Design review of the part built by this model. Coordinates are the model's own, in mm. Give positions to 0.01 mm unless a question says otherwise; leave off trailing zeros. Loops run counter-clockwise (first coordinate to the right, second up) from the corner with the lowest first, then second, coordinate; pieces in that order, holes last.
from build123d import *

# Parameters (mm, degrees)
SKETCH_1_W             = 0.8
SKETCH_1_H             = 15
EXTRUDE_1_DEPTH        = 203
SKETCH_2_R             = 2.5
SKETCH_3_R             = 1.5
CUT_EXTRUDE_1_DEPTH    = 407.407738607
SKETCH_10_W            = 33
SKETCH_10_H            = 6
CUT_EXTRUDE_4_DEPTH    = 60
PATTERN_LINEAR_1_COUNT = 8
PATTERN_LINEAR_1_PITCH = 50


with BuildPart() as part:
    # 草图1 → 拉伸-薄壁1 (new, symmetric)
    with BuildSketch(Plane.XY):
        with Locations((0.4, 7.5)):
            Rectangle(SKETCH_1_W, SKETCH_1_H)
    extrude(amount=EXTRUDE_1_DEPTH, both=True)

    # 扫描1: sweep along a curve in space
    with BuildLine() as sweep_1_path:
        Line((0.8, 15, 203), (0.8, 15, -203))
    # 草图2 → 扫描1 (sweep)
    with BuildSketch(Plane.XY.offset(203)):
        with Locations((2.5, 15)):
            Circle(SKETCH_2_R)
    sweep(path=sweep_1_path.line)

    # 草图3 → 切除-拉伸1 (cut, through all)
    with BuildSketch(Plane.XY.offset(203)):
        with Locations((2.5, 15)):
            Circle(SKETCH_3_R)
    extrude(amount=-CUT_EXTRUDE_1_DEPTH, mode=Mode.SUBTRACT)

    # 草图10 → 切除-拉伸4 (cut, symmetric)
    with BuildSketch(Plane(origin=(0.8, 0, 0), x_dir=(0, 0, -1), z_dir=(1, 0, 0))):
        with Locations((-165, 15)):
            Rectangle(SKETCH_10_W, SKETCH_10_H)
        with Locations((-99, 15)):
            Rectangle(SKETCH_10_W, SKETCH_10_H)
        with Locations((-33, 15)):
            Rectangle(SKETCH_10_W, SKETCH_10_H)
        with Locations((33, 15)):
            Rectangle(SKETCH_10_W, SKETCH_10_H)
        with Locations((99, 15)):
            Rectangle(SKETCH_10_W, SKETCH_10_H)
        with Locations((165, 15)):
            Rectangle(SKETCH_10_W, SKETCH_10_H)
    extrude(amount=CUT_EXTRUDE_4_DEPTH, both=True, mode=Mode.SUBTRACT)

    # 草图12 → M3 锥坑平头螺钉的锥形沉头孔2 (revolve, cut)
    with BuildSketch(Plane(origin=(0.8, 5.5, -175), x_dir=(0, 0, -1), z_dir=(0, 1, 0))):
        Polygon((0, 0), (0, 0.8), (1.7, 0.8), (1.7, 1.45), (3.15, 0), align=None)
    hole_wizard_m3_2 = revolve(axis=Axis((7.15, 5.5, -175), (-1, 0, 0)), mode=Mode.SUBTRACT)

    # 阵列(线性)1: M3 锥坑平头螺钉的锥形沉头孔2 ×8
    with Locations(*[(0, 0, i * PATTERN_LINEAR_1_PITCH) for i in range(1, PATTERN_LINEAR_1_COUNT)]):
        add(hole_wizard_m3_2, mode=Mode.SUBTRACT)


solid = part.part
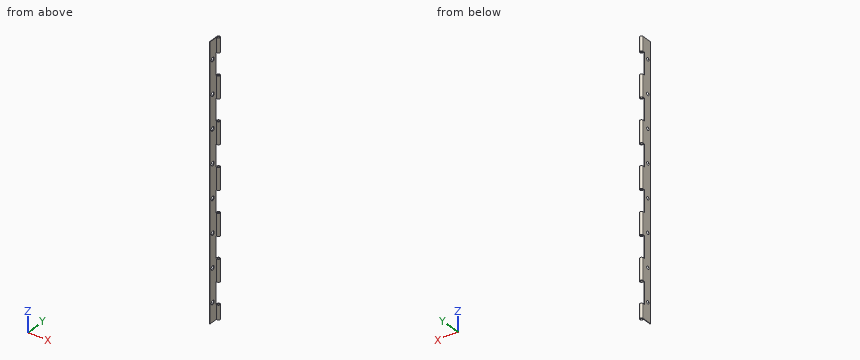
Q1. Take a section at B-B (z = -97). Give the boundary of the cut face in (x, y), plus the area to 3 significant figures.
Results:
outline: (0, 0) - (0.8, 0) - (0.8, 12) - (0, 12) - close
area: 9.60 mm2
Q2. Insertion check: pin 1 (0.9 mm diameter, centred on x = 0.5, z = -160, fed in from +Y); pin 2 (2 mm diameter, centred on x = 4.5, z = 118, fed in from +Y); pin 3 (2 mm diameter, centred on y = 6.5, z = 103.5, fed in from +X). Each pin has a flat end and moves straight along its axis. Give the tip position at first contact, or say it passes through.
Results:
pin 1: stops at y = 12
pin 2: stops at y = 17.29
pin 3: stops at x = 0.8
Q3. Take a section at A-A (y = 5.5). Give the number of separate pieces and of enclosed holes in the cut face, plus the area to 3 significant figures.
Results:
separate pieces: 9
enclosed holes: 0
area: 290 mm2
Q4. Wall thickness on line 1 (Y direction, x = 2.5, z = 124); line 2 (X direction, y = 10.75, z = 140); line 3 (Y direction, x = 4.3, z = 78): over which ranges is each line inside the solid? List them lowest first.
Results:
line 1: y = 12.5 to 13.5, 16.5 to 17.5
line 2: x = 0 to 0.8
line 3: y = 13.27 to 16.73
